```python
from build123d import *

# Parameters (mm, degrees)
F0_R     = 76.2
F1_DEPTH = 6.35


with BuildPart() as f1:
    # F0 (on Top) → F1 (new body)
    with BuildSketch(Plane.XY):
        Circle(F0_R)
        with BuildLine():
            Line((-3.175, -25.4), (-3.175, -3.175))
            Line((-3.175, -3.175), (-25.4, -3.175))
            ThreePointArc((-25.4, -3.175), (-28.575, 0), (-25.4, 3.175))
            Line((-25.4, 3.175), (-3.175, 3.175))
            Line((-3.175, 3.175), (-3.175, 25.4))
            ThreePointArc((-3.175, 25.4), (0, 28.575), (3.175, 25.4))
            Line((3.175, 25.4), (3.175, 3.175))
            Line((3.175, 3.175), (25.4, 3.175))
            ThreePointArc((25.4, 3.175), (28.575, 0), (25.4, -3.175))
            Line((25.4, -3.175), (3.175, -3.175))
            Line((3.175, -3.175), (3.175, -25.4))
            ThreePointArc((3.175, -25.4), (0, -28.575), (-3.175, -25.4))
        make_face(mode=Mode.SUBTRACT)
    extrude(amount=F1_DEPTH)


solid = f1.part
```
Build history of the part. All positions in model axes, mm. Coordinates: 2 decimals unless noted, no trailing zeros. Write each loop counter-clockwise with the first axis right and the second up, starting at its lowest first coordinate (ties: lowest second). Pieces come first, ordered by that corner, then holes.
1. Band-saw the part on D-D, the plane x = 42. Give the cut face in (y, z), and give its area (3 significant figures).
Answer block:
outline: (-63.58, 0) - (63.58, 0) - (63.58, 6.35) - (-63.58, 6.35) - close
area: 807 mm2
2. Band-saw the part on B-B, the plane x = 0. Give the cut face in (y, z) (3 decimals), and give its area (3 significant figures).
Answer block:
outline: (-76.2, 0) - (-28.575, 0) - (-28.575, 6.35) - (-76.2, 6.35) - close; (28.575, 0) - (76.2, 0) - (76.2, 6.35) - (28.575, 6.35) - close
area: 605 mm2
3. Drill centre lines: probe 1 along X at (y, z) = (-26, 2.25); probe 2 along Y at (x, z) = (16.5, 2) (3 decimals); probe 3 along X at (y, z) = (-24, 2.25) (3 decimals). Where is each one in solid material? Low to high.
Answer block:
probe 1: x = -71.63 to -3.12, 3.12 to 71.63
probe 2: y = -74.392 to -3.175, 3.175 to 74.392
probe 3: x = -72.322 to -3.175, 3.175 to 72.322
4. Drop flat-ended pins along their axis: pin 1 (1 mm diameter, centred on x = 27.5, z = 2.5, fed in from -Y); pin 2 (3 mm diameter, centred on x = -19.5, z = 2, fed in from -Y); pin 3 (3 mm diameter, centred on y = -53.5, z = 1, fed in from -X). Give the stop position or say it passes through.
Answer block:
pin 1: stops at y = -71.26
pin 2: stops at y = -74.04
pin 3: stops at x = -55.7
5. Band-saw the part on A-A, the plane z = 4.5. Give the cut face in (x, y) (3 decimals).
Answer block:
outline: circle Ø152.4 at (0, 0); hole (-25.4, -3.175) - (-3.175, -3.175) - (-3.175, -25.4) arc R3.175 ccw to (3.175, -25.4) - (3.175, -3.175) - (25.4, -3.175) arc R3.175 ccw to (25.4, 3.175) - (3.175, 3.175) - (3.175, 25.4) arc R3.175 ccw to (-3.175, 25.4) - (-3.175, 3.175) - (-25.4, 3.175) arc R3.175 ccw to start
6. Pull direction Z, two halves, no side cores. Call faces 1 (the flat face through (14, -3.175, 3)), 2 (the flat face through (16, -16, 6.35)), 3 (the flat face through (16, -16, 0)): released by +Z, released by -Z, zero draft, split by the parting line, or undercut.
Answer block:
face 1: zero draft
face 2: released by +Z
face 3: released by -Z
